from build123d import *

# Parameters (mm, degrees)
F1_DEPTH = 63.5
F2_DEPTH = 25.4
F3_DEPTH = 7.9375
F5_R     = 6.35


with BuildPart() as f1:
    # F0 (on Front) → F1 (new body, symmetric)
    with BuildSketch(Plane.XZ):
        Polygon((-41.275, -9.525), (41.275, -9.525), (41.275, 9.525), (22.225, 9.525), (-41.275, 9.525), align=None)
    extrude(amount=F1_DEPTH, both=True)

    # F0 (on Front) → F2 (join, symmetric)
    with BuildSketch(Plane.XZ):
        with BuildLine():
            Line((22.225, 9.525), (41.275, 9.525))
            Line((41.275, 9.525), (41.275, 27.0002))
            ThreePointArc((41.275, 27.0002), (45.92468, 38.22552), (57.15, 42.8752))
            Line((57.15, 42.8752), (58.186395, 42.8752))
            Line((58.186395, 42.8752), (58.186395, 61.846107))
            add(Edge.make_bspline(
                [(54.311995, 61.809701), (55.594718, 61.823662), (56.886272, 61.835647), (58.186395, 61.846107)],
                knots=[110.184899, 110.184899, 110.184899, 110.184899, 112.679002, 112.679002, 112.679002, 112.679002], degree=3))
            ThreePointArc((54.311995, 61.809701), (31.470505, 50.671261), (22.225, 27.0002))
            Line((22.225, 27.0002), (22.225, 9.525))
        make_face()
    extrude(amount=F2_DEPTH, both=True)

    # F0 (on Front) → F3 (join, symmetric)
    with BuildSketch(Plane.XZ):
        with BuildLine():
            add(Edge.make_bspline(
                [(-41.275, 9.525), (-41.788435, 56.718878), (-2.356346, 61.192912), (54.311995, 61.809701)],
                knots=[0, 0, 0, 0, 110.184899, 110.184899, 110.184899, 110.184899], degree=3))
            Line((-41.275, 9.525), (22.225, 9.525))
            Line((22.225, 9.525), (22.225, 27.0002))
            ThreePointArc((22.225, 27.0002), (31.470505, 50.671261), (54.311995, 61.809701))
        make_face()
    extrude(amount=F3_DEPTH, both=True)

    # F0 (on Front) → F4 (revolve)
    with BuildSketch(Plane.XZ):
        Polygon((82.170509, 61.855137), (82.170509, 42.8752), (82.170509, 38.1), (108.986395, 38.1), (108.986395, 66.675), (82.170509, 66.675), align=None)
    revolve(axis=Axis((82.170509, 0, 51.389013), (0, 0, -1)))

    # F5
    f5_edges = [f1.edges().sort_by_distance(p)[0] for p in [
        (41.275, -63.5, 0),
        (-41.275, -63.5, 0),
        (41.275, 63.5, 0),
        (-41.275, 63.5, 0),
    ]]
    fillet(f5_edges, radius=F5_R)


solid = f1.part
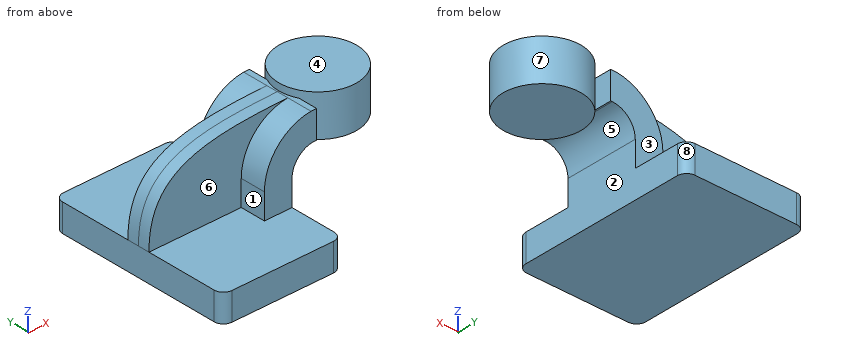
Here's how the part is built. I have some questions about the finished solid (model axes, mm). Face numbers are marked on the shaded views. A direction names the side the tool comes from. Round coordinates to 2 decimals unless told otherwise and drop trailing zeros. Loops run counter-clockwise (first coordinate to the right, second up) from the corner with the lowest first, then second, coordinate; pieces in that order, holes last.
1. Which directions (+Z, -Z, +X, -X, +Y, -Y) give clear straight access to the entire face, cutting with the end or side of a thin tool? Please do the marked faces 1, 2, 3 and 4.
Answer list:
face 1: +Z, -X, -Y
face 2: -Z, +X, +Y, -Y
face 3: +Z, -X, +Y
face 4: +Z, +X, -X, +Y, -Y
2. If I drill on line 1 along Z through (x, y) = (-27, -18.5) (3 decimals); line 2 along X through (y, z) = (4, 4) (3 decimals); line 3 along Y through (x, z) = (-34, 33.5), over which ranges is the centre line in solid material (lowest first)?
Answer list:
line 1: z = -9.525 to 9.525
line 2: x = -41.275 to 41.275
line 3: y = -7.94 to 7.94
3. If we section it at B-B on x = 95.5: Write out the boundary of the cut face in (y, z) (3 decimals), plus the area to 3 significant figures.
Answer list:
outline: (-23.268, 38.1) - (23.268, 38.1) - (23.268, 66.675) - (-23.268, 66.675) - close
area: 1,330 mm2
4. For P1, Ø10.5, axis at y = -15.5, z = 49.5, coming from the +X side; P2, Ø8, axis at x = -24.5, y = 28, coming from the +Z side (3 decimals); P3, Ø10, axis at x = 67.5, z = 54, coming from the +Y side, each with a flat end and sliding along its axis, tell me the tip position at first contact or that it passes through.
Answer list:
P1: stops at x = 106.95
P2: stops at z = 9.525
P3: stops at y = 25.01
5. If we section it at A-A on y = 43.5: Write out the boundary of the cut face in (x, z) (3 decimals), plus the area to 3 significant figures.
Answer list:
outline: (-41.275, -9.525) - (41.275, -9.525) - (41.275, 9.525) - (-41.275, 9.525) - close
area: 1,570 mm2
6. We'd pull the mould along X, two halves only. Please class the marked faces 5, 6, 7 and 8: +X half, -X half, draft (parallel to the pull), parting line (faces both ways), or undercut.
Answer list:
face 5: undercut
face 6: draft
face 7: undercut
face 8: +X half
